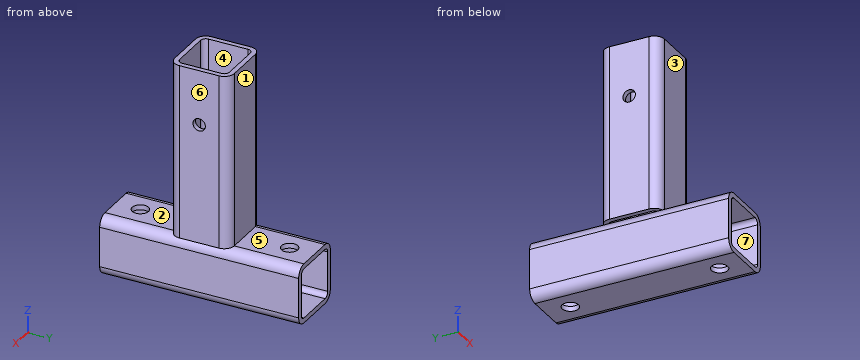
```python
from build123d import *

# Parameters (mm, degrees)
F1_DEPTH = 87.5
F3_DEPTH = 100
F4_R     = 8.25
F5_DEPTH = 60.001
F6_R     = 6.25
F7_DEPTH = 60.001


with BuildPart() as f1:
    # F0 (on Top) → F1 (new body, symmetric)
    with BuildSketch(Plane.XY):
        with BuildLine():
            Line((20, 30), (-20, 30))
            ThreePointArc((-20, 30), (-27.071068, 27.071068), (-30, 20))
            Line((-30, 20), (-30, -20))
            ThreePointArc((-30, -20), (-27.071068, -27.071068), (-20, -30))
            Line((-20, -30), (20, -30))
            ThreePointArc((20, -30), (27.071068, -27.071068), (30, -20))
            Line((30, -20), (30, 20))
            ThreePointArc((30, 20), (27.071068, 27.071068), (20, 30))
        make_face()
        with BuildLine():
            ThreePointArc((-25, 20), (-23.535534, 23.535534), (-20, 25))
            Line((-20, 25), (20, 25))
            ThreePointArc((20, 25), (23.535534, 23.535534), (25, 20))
            Line((25, 20), (25, -20))
            ThreePointArc((25, -20), (23.535534, -23.535534), (20, -25))
            Line((20, -25), (-20, -25))
            ThreePointArc((-20, -25), (-23.535534, -23.535534), (-25, -20))
            Line((-25, -20), (-25, 20))
        make_face(mode=Mode.SUBTRACT)
    extrude(amount=F1_DEPTH, both=True)

    # F2 (on Front) → F3 (join, symmetric)
    with BuildSketch(Plane.XZ):
        with BuildLine():
            Line((20, -87.5), (-20, -87.5))
            ThreePointArc((-20, -87.5), (-27.071068, -90.428932), (-30, -97.5))
            Line((-30, -97.5), (-30, -137.5))
            ThreePointArc((-30, -137.5), (-27.071068, -144.571068), (-20, -147.5))
            Line((-20, -147.5), (20, -147.5))
            ThreePointArc((20, -147.5), (27.071068, -144.571068), (30, -137.5))
            Line((30, -137.5), (30, -97.5))
            ThreePointArc((30, -97.5), (27.071068, -90.428932), (20, -87.5))
        make_face()
        with BuildLine():
            ThreePointArc((20, -92.5), (23.535534, -93.964466), (25, -97.5))
            Line((25, -97.5), (25, -137.5))
            ThreePointArc((25, -137.5), (23.535534, -141.035534), (20, -142.5))
            Line((20, -142.5), (-20, -142.5))
            ThreePointArc((-20, -142.5), (-23.535534, -141.035534), (-25, -137.5))
            Line((-25, -137.5), (-25, -97.5))
            ThreePointArc((-25, -97.5), (-23.535534, -93.964466), (-20, -92.5))
            Line((-20, -92.5), (20, -92.5))
        make_face(mode=Mode.SUBTRACT)
    extrude(amount=F3_DEPTH, both=True)

    # F4 (on face) → F5 (cut, through all)
    with BuildSketch(Plane.XY.offset(-87.5)):
        with Locations((0, 75)):
            Circle(F4_R)
        with Locations((0, -75)):
            Circle(F4_R)
    extrude(amount=-F5_DEPTH, mode=Mode.SUBTRACT)

    # F6 (on face) → F7 (cut, through all)
    with BuildSketch(Plane.YZ.offset(30)):
        with Locations((0, 32.5)):
            Circle(F6_R)
    extrude(amount=-F7_DEPTH, mode=Mode.SUBTRACT)


solid = f1.part
```
Design review of the part built by this model. Coordinates are the model's own, in mm. Face numbers are marked on the shaded views. A direction names the side the tool comes from. Give positions to 0.01 mm unless a question says otherwise; leave off trailing zeros. Order: outer loops, then holes, each group sorted by start corner. A loop starts at its lowest first (then second) coordinate and runs counter-clockwise, first axis right, second up. Notation, with made-up numbers: (-39, -28) -> (-25, -28) arc R22 ccw to (-25, -9) -> close; hole circle Ø3 at (-4.75, 71). An arc over 180 degrees is marked (long way). Write each question's results on one line, items separated by ' | '. Start each with the question number.
Q1. Add section D-D on y = -75. Give the boundary of the cut face in (x, z), and give its area (3 significant figures).
Q2. Add section B-B on x = -17. Give the boundary of the cut face in (y, z).
Q3. Machinability: for the marked faces 5, 6 and 7, which of the approach directions +Z, -Z, +X, -X, +Y, -Y give a long, thin tool a straight path to every point of the face, cutting with its end or side? Answer none if there is none.
Q4. Mouldability with a two-part tool opening along Y and no side actions: class the marked faces 1, 2, 3 and 4 as +Y half, -Y half, draft (parallel to the pull), parting line (faces both ways), or undercut.
Q5. Add section C-C on z = -128.5. Give the boundary of the cut face in (x, y), and give its area (3 significant figures).
Q6. Add section A-A on y = 16. Give the boundary of the cut face in (x, z), and give its area (3 significant figures).
Q7. For pin 1 (5 mm diameter, centred on x = -23, y = 11, fed in from -Z); pin 2 (10 mm diameter, centred on x = 4.5, y = 19, fed in from +Z); pin 3 (12 mm diameter, centred on x = -8.5, z = 9, fed in from -Y); pin 4 (11 mm diameter, centred on y = 0, z = 32.5, fed in from +X), all flat-tipped, find the tip position at first contact; note any pin that passes through.
Q8. Wall thickness on L1, parallel to Y at x = 0, z = -144.9; L2, parallel to Z at x = -3, y = 30.5; L3, parallel to Y at x = 15, z = -7: over which ranges is each line inside the solid? List them lowest first. Write a range as from..to.
Found:
1) outline: (-30, -137.5) arc R10 ccw to (-20, -147.5) -> (-8.25, -147.5) -> (-8.25, -142.5) -> (-20, -142.5) arc R5 cw to (-25, -137.5) -> (-25, -97.5) arc R5 cw to (-20, -92.5) -> (-8.25, -92.5) -> (-8.25, -87.5) -> (-20, -87.5) arc R10 ccw to (-30, -97.5) -> close; (8.25, -147.5) -> (20, -147.5) arc R10 ccw to (30, -137.5) -> (30, -97.5) arc R10 ccw to (20, -87.5) -> (8.25, -87.5) -> (8.25, -92.5) -> (20, -92.5) arc R5 cw to (25, -97.5) -> (25, -137.5) arc R5 cw to (20, -142.5) -> (8.25, -142.5) -> close | area: 871 mm2
2) outline: (-100, -147.5) -> (100, -147.5) -> (100, -142.5) -> (-100, -142.5) -> close; (-100, -92.5) -> (100, -92.5) -> (100, -87.5) -> (30, -87.5) -> (30, 87.5) -> (25, 87.5) -> (25, -87.5) -> (-25, -87.5) -> (-25, 87.5) -> (-30, 87.5) -> (-30, -87.5) -> (-100, -87.5) -> close
3) face 5: +Z, +X, -X, +Y | face 6: +Z, -Z, +X, +Y, -Y | face 7: +Y, -Y
4) face 1: +Y half | face 2: draft | face 3: -Y half | face 4: undercut
5) outline: (-30, -100) -> (-25, -100) -> (-25, 100) -> (-30, 100) -> close; (25, -100) -> (30, -100) -> (30, 100) -> (25, 100) -> close | area: 2,000 mm2
6) outline: (-30, -137.5) arc R10 ccw to (-20, -147.5) -> (20, -147.5) arc R10 ccw to (30, -137.5) -> (30, -97.5) arc R10 ccw to (20, -87.5) -> (-20, -87.5) arc R10 ccw to (-30, -97.5) -> close; (-30, -87.5) -> (-25, -87.5) -> (-25, 87.5) -> (-30, 87.5) -> close; (25, -87.5) -> (30, -87.5) -> (30, 87.5) -> (25, 87.5) -> close; hole (-25, -137.5) arc R5 ccw to (-20, -142.5) -> (20, -142.5) arc R5 ccw to (25, -137.5) -> (25, -97.5) arc R5 ccw to (20, -92.5) -> (-20, -92.5) arc R5 ccw to (-25, -97.5) -> close | area: 2,790 mm2
7) pin 1: stops at z = -147.49 | pin 2: stops at z = -87.5 | pin 3: stops at y = -30 | pin 4: passes through
8) L1: y = -100..-83.25, -66.75..66.75, 83.25..100 | L2: z = -147.5..-142.5, -92.5..-87.5 | L3: y = -30..-25, 25..30
